from build123d import *

# Parameters (mm, degrees)
F1_DEPTH = 3.175
F2_W     = 3.175
F2_H     = 38.1
F3_DEPTH = 19.05


with BuildPart() as f1:
    # F0 (on Top) → F1 (new body)
    with BuildSketch(Plane.XY):
        with BuildLine():
            Line((0, 10.6418100238), (0, 29.6918100238))
            Line((0, 29.6918100238), (-7.9375, 29.6918100238))
            ThreePointArc((-7.9375, 29.6918100238), (-9.525, 28.1043100238), (-11.1125, 29.6918100238))
            Line((-11.1125, 29.6918100238), (-12.7, 29.6918100238))
            ThreePointArc((-12.7, 29.6918100238), (-13.1833649686, 27.2617702283), (-14.5598719395, 25.2016819633))
            Line((-14.5598719395, 25.2016819633), (-13.4373399243, 24.0791499481))
            ThreePointArc((-13.4373399243, 24.0791499481), (-11.7072979603, 24.4232766908), (-10.7273079092, 22.956617933))
            ThreePointArc((-10.7273079092, 22.956617933), (-10.8481491513, 22.3491079841), (-11.1922758941, 21.8340859178))
            Line((-11.1922758941, 21.8340859178), (-8.0172758941, 18.6590859178))
            ThreePointArc((-8.0172758941, 18.6590859178), (-6.2872339301, 19.0032126606), (-5.3072438789, 17.5365539027))
            ThreePointArc((-5.3072438789, 17.5365539027), (-5.4280851211, 16.9290439538), (-5.7722118638, 16.4140218876))
            Line((-5.7722118638, 16.4140218876), (0, 10.6418100238))
        make_face()
        with BuildLine():
            Line((-19.05, 18.5793100238), (-19.05, 10.6418100238))
            Line((-19.05, 10.6418100238), (0, 10.6418100238))
            Line((0, 10.6418100238), (-5.7722118638, 16.4140218876))
            ThreePointArc((-5.7722118638, 16.4140218876), (-8.0172758941, 16.4140218876), (-8.0172758941, 18.6590859178))
            Line((-8.0172758941, 18.6590859178), (-11.1922758941, 21.8340859178))
            ThreePointArc((-11.1922758941, 21.8340859178), (-13.4373399243, 21.8340859178), (-13.4373399243, 24.0791499481))
            Line((-13.4373399243, 24.0791499481), (-14.5598719395, 25.2016819633))
            ThreePointArc((-14.5598719395, 25.2016819633), (-16.6199602045, 23.8251749923), (-19.05, 23.3418100238))
            Line((-19.05, 23.3418100238), (-19.05, 21.7543100238))
            ThreePointArc((-19.05, 21.7543100238), (-17.9274679849, 21.2893420389), (-17.4625, 20.1668100238))
            ThreePointArc((-17.4625, 20.1668100238), (-17.9274679849, 19.0442780087), (-19.05, 18.5793100238))
        make_face()
        with BuildLine():
            Line((-31.3978521665, 17.3439578573), (-38.1, 10.6418100238))
            Line((-38.1, 10.6418100238), (-19.05, 10.6418100238))
            Line((-19.05, 10.6418100238), (-19.05, 18.5793100238))
            ThreePointArc((-19.05, 18.5793100238), (-20.6375, 20.1668100238), (-19.05, 21.7543100238))
            Line((-19.05, 21.7543100238), (-19.05, 23.3418100238))
            ThreePointArc((-19.05, 23.3418100238), (-21.4800397955, 23.8251749923), (-23.5401280605, 25.2016819632))
            Line((-23.5401280605, 25.2016819633), (-24.6626600757, 24.0791499481))
            ThreePointArc((-24.6626600757, 24.0791499481), (-24.3185333329, 23.5641278819), (-24.1976920908, 22.956617933))
            ThreePointArc((-24.1976920908, 22.956617933), (-25.1776821419, 21.4899591751), (-26.9077241059, 21.8340859178))
            Line((-26.9077241059, 21.8340859178), (-29.1527881362, 19.5890218876))
            ThreePointArc((-29.1527881362, 19.5890218876), (-28.8086613935, 19.0739998213), (-28.6878201513, 18.4664898724))
            ThreePointArc((-28.6878201513, 18.4664898724), (-29.6678102025, 16.9998311146), (-31.3978521665, 17.3439578573))
        make_face()
        with BuildLine():
            Line((-30.1625, 29.6918100238), (-38.1, 29.6918100238))
            Line((-38.1, 29.6918100238), (-38.1, 10.6418100238))
            Line((-38.1, 10.6418100238), (-31.3978521665, 17.3439578573))
            ThreePointArc((-31.3978521665, 17.3439578573), (-31.3978521665, 19.5890218876), (-29.1527881362, 19.5890218876))
            Line((-29.1527881362, 19.5890218876), (-26.9077241059, 21.8340859178))
            ThreePointArc((-26.9077241059, 21.8340859178), (-26.9077241059, 24.0791499481), (-24.6626600757, 24.0791499481))
            Line((-24.6626600757, 24.0791499481), (-23.5401280605, 25.2016819633))
            ThreePointArc((-23.5401280605, 25.2016819632), (-24.9166350314, 27.2617702283), (-25.4, 29.6918100238))
            Line((-25.4, 29.6918100238), (-26.9875, 29.6918100238))
            ThreePointArc((-26.9875, 29.6918100238), (-28.575, 28.1043100238), (-30.1625, 29.6918100238))
        make_face()
        with BuildLine():
            Line((-31.3978521665, 42.0396621903), (-38.1, 48.7418100238))
            Line((-38.1, 48.7418100238), (-38.1, 29.6918100238))
            Line((-38.1, 29.6918100238), (-30.1625, 29.6918100238))
            ThreePointArc((-30.1625, 29.6918100238), (-28.575, 31.2793100238), (-26.9875, 29.6918100238))
            Line((-26.9875, 29.6918100238), (-25.4, 29.6918100238))
            ThreePointArc((-25.4, 29.6918100238), (-24.9166350314, 32.1218498193), (-23.5401280605, 34.1819380843))
            Line((-23.5401280605, 34.1819380843), (-24.6626600757, 35.3044700995))
            ThreePointArc((-24.6626600757, 35.3044700995), (-26.9077241059, 35.3044700995), (-26.9077241059, 37.5495341297))
            Line((-26.9077241059, 37.5495341297), (-29.1527881362, 39.79459816))
            ThreePointArc((-29.1527881362, 39.79459816), (-31.3978521665, 39.79459816), (-31.3978521665, 42.0396621903))
        make_face()
        with BuildLine():
            Line((-19.05, 48.7418100238), (-38.1, 48.7418100238))
            Line((-38.1, 48.7418100238), (-31.3978521665, 42.0396621903))
            ThreePointArc((-31.3978521665, 42.0396621903), (-29.6678102025, 42.383788933), (-28.6878201513, 40.9171301751))
            ThreePointArc((-28.6878201513, 40.9171301751), (-28.8086613935, 40.3096202262), (-29.1527881362, 39.79459816))
            Line((-29.1527881362, 39.79459816), (-26.9077241059, 37.5495341297))
            ThreePointArc((-26.9077241059, 37.5495341297), (-25.1776821419, 37.8936608724), (-24.1976920908, 36.4270021146))
            ThreePointArc((-24.1976920908, 36.4270021146), (-24.3185333329, 35.8194921657), (-24.6626600757, 35.3044700995))
            Line((-24.6626600757, 35.3044700995), (-23.5401280605, 34.1819380843))
            ThreePointArc((-23.5401280605, 34.1819380843), (-21.4800397955, 35.5584450552), (-19.05, 36.0418100238))
            Line((-19.05, 36.0418100238), (-19.05, 37.6293100238))
            ThreePointArc((-19.05, 37.6293100238), (-20.6375, 39.2168100238), (-19.05, 40.8043100238))
            Line((-19.05, 40.8043100238), (-19.05, 48.7418100238))
        make_face()
        with BuildLine():
            Line((0, 48.7418100238), (-19.05, 48.7418100238))
            Line((-19.05, 48.7418100238), (-19.05, 40.8043100238))
            ThreePointArc((-19.05, 40.8043100238), (-17.9274679849, 40.3393420389), (-17.4625, 39.2168100238))
            ThreePointArc((-17.4625, 39.2168100238), (-17.9274679849, 38.0942780087), (-19.05, 37.6293100238))
            Line((-19.05, 37.6293100238), (-19.05, 36.0418100238))
            ThreePointArc((-19.05, 36.0418100238), (-16.6199602045, 35.5584450552), (-14.5598719395, 34.1819380843))
            Line((-14.5598719395, 34.1819380843), (-13.4373399243, 35.3044700995))
            ThreePointArc((-13.4373399243, 35.3044700995), (-13.4373399243, 37.5495341297), (-11.1922758941, 37.5495341297))
            Line((-11.1922758941, 37.5495341297), (-8.9472118638, 39.79459816))
            ThreePointArc((-8.9472118638, 39.79459816), (-8.9472118638, 42.0396621903), (-6.7021478335, 42.0396621903))
            Line((-6.7021478335, 42.0396621903), (0, 48.7418100238))
        make_face()
        with BuildLine():
            Line((0, 29.6918100238), (0, 48.7418100238))
            Line((0, 48.7418100238), (-6.7021478335, 42.0396621903))
            ThreePointArc((-6.7021478335, 42.0396621903), (-6.3580210908, 41.524640124), (-6.2371798487, 40.9171301751))
            ThreePointArc((-6.2371798487, 40.9171301751), (-7.2171698998, 39.4504714173), (-8.9472118638, 39.79459816))
            Line((-8.9472118638, 39.79459816), (-11.1922758941, 37.5495341297))
            ThreePointArc((-11.1922758941, 37.5495341297), (-10.8481491513, 37.0345120635), (-10.7273079092, 36.4270021146))
            ThreePointArc((-10.7273079092, 36.4270021146), (-11.7072979603, 34.9603433567), (-13.4373399243, 35.3044700995))
            Line((-13.4373399243, 35.3044700995), (-14.5598719395, 34.1819380843))
            ThreePointArc((-14.5598719395, 34.1819380843), (-13.1833649686, 32.1218498193), (-12.7, 29.6918100238))
            Line((-12.7, 29.6918100238), (-11.1125, 29.6918100238))
            ThreePointArc((-11.1125, 29.6918100238), (-9.525, 31.2793100238), (-7.9375, 29.6918100238))
            Line((-7.9375, 29.6918100238), (0, 29.6918100238))
        make_face()
    extrude(amount=F1_DEPTH)

    # F2 (on face) → F3 (join)
    with BuildSketch(Plane.XY.offset(3.175)):
        with Locations((-1.5875, 29.6918100238)):
            Rectangle(F2_W, F2_H)
    extrude(amount=F3_DEPTH)


solid = f1.part
Check sheet for the modelled part. Datum: model origin and axes. Units: mm. A direction names the side the tool comes from. Round coordinates to 2 decimals unless told otherwise and drop trailing zeros. Order: outer loops, then holes, each group sorted by start corner. A loop starts at its lowest first (then second) coordinate and runs counter-clockwise, first axis right, second up.
Q1. Cross-section at B-B, the plane x = -28. Enter the section's corners in (y, z) (3 decimals).
Filled sheet:
outline: (10.642, 0) - (28.212, 0) - (28.212, 3.175) - (10.642, 3.175) - close; (31.172, 0) - (48.742, 0) - (48.742, 3.175) - (31.172, 3.175) - close
Q2. Cross-section at C-C, the plane z = 2. Give the number of separate pieces and of enclosed holes in the cut face, plus the area to 3 significant figures.
Filled sheet:
separate pieces: 1
enclosed holes: 13
area: 1,230 mm2
Q3. Set-up check for faces 1 (the face through (-38.1, 30, 2)), 2 (the face through (-25, 34, 3.175)): record each of +Z, -Z, +X, -X, +Y, -Y from which the full face is reachable in a straight line by a thin tool's end or side.
Filled sheet:
face 1: +Z, -Z, -X, +Y, -Y
face 2: +Z, -X, +Y, -Y
Q4. Draft check along Y on faces 3 (the face through (-9.181, 28.142, 1.565)), 4 (the face through (-13, 10.642, 3)), 5 (the face through (-24, 34, 0)). Enter one of: pulls with the +Y half, pulls with the -Y half, needs draft (parallel to the pull), parting line crosses it, or undercut.
Filled sheet:
face 3: undercut
face 4: pulls with the -Y half
face 5: needs draft
Q5. Cross-section at D-D, the plane y = 46.5. Enter the section's corners in (x, z) (3 decimals).
Filled sheet:
outline: (-38.1, 0) - (0, 0) - (0, 22.225) - (-3.175, 22.225) - (-3.175, 3.175) - (-38.1, 3.175) - close
Q6. Scan lines: L1, parallel to X at y = 32, z = 18.75 (3 decimals); L2, parallel to Z at x = -34, y = 31.5 (3 decimals). Record each from-to range of solid material in increasing order.
Filled sheet:
L1: x = -3.175 to 0
L2: z = 0 to 3.175
Q7. Depth check by flat-ended pin: P1, Ø12, axis at y = 40, z = 5, coming from the -X side; P2, Ø10.5, axis at x = -15, y = 35.5, coming from the +Z side (3 decimals); P3, Ø6, axis at x = -17.5, y = 28.5, coming from the -Z side. Enter the tip coordinate at first touch or a pass-through.
Filled sheet:
P1: stops at x = -38.1
P2: stops at z = 3.175
P3: passes through
Q8. Cross-section at A-A, the plane y = 30.5. Enter the section's corners in (x, z) (3 decimals), plus the area to 3 significant figures.
Filled sheet:
outline: (-38.1, 0) - (-29.941, 0) - (-29.941, 3.175) - (-38.1, 3.175) - close; (-27.209, 0) - (-25.348, 0) - (-25.348, 3.175) - (-27.209, 3.175) - close; (-12.752, 0) - (-10.891, 0) - (-10.891, 3.175) - (-12.752, 3.175) - close; (-8.159, 0) - (0, 0) - (0, 22.225) - (-3.175, 22.225) - (-3.175, 3.175) - (-8.159, 3.175) - close
area: 124 mm2
